Read the model definition and answer for the solid it produces. Units are mm, in the model's axes. Give positions to 0.01 mm unless a question says otherwise; leave off trailing zeros. Write each loop counter-clockwise with the first axis right and the second up, starting at its lowest first coordinate (ties: lowest second). Pieces come first, ordered by that corner, then holes. Notation, with made-up numbers: (71, 32) -> (87, 32) arc R21 cw to (87, 61) -> close; hole circle Ø3 at (46.5, 14.5). An arc over 180 degrees is marked (long way). Use a Markdown table: item, result.
from build123d import *

# Parameters (mm, degrees)
MAIN_PROFILE_SKETCH_W = 70
MAIN_PROFILE_SKETCH_H = 106
MAIN_PROFILE_SKETCH_R = 1.7
MAIN_EXTRUSION_DEPTH  = 3


with BuildPart() as part:
    # Main Profile Sketch → Main Extrusion (new body)
    with BuildSketch(Plane.XY.offset(88)):
        with Locations((-203, 0)):
            Rectangle(MAIN_PROFILE_SKETCH_W, MAIN_PROFILE_SKETCH_H)
        with Locations((-234, -51)):
            Circle(MAIN_PROFILE_SKETCH_R, mode=Mode.SUBTRACT)
        with Locations((-221, -39)):
            Circle(MAIN_PROFILE_SKETCH_R, mode=Mode.SUBTRACT)
        with Locations((-221, -25)):
            Circle(MAIN_PROFILE_SKETCH_R, mode=Mode.SUBTRACT)
        with Locations((-224, -5)):
            Circle(MAIN_PROFILE_SKETCH_R, mode=Mode.SUBTRACT)
        with Locations((-210, -5)):
            Circle(MAIN_PROFILE_SKETCH_R, mode=Mode.SUBTRACT)
        with Locations((-172, -51)):
            Circle(MAIN_PROFILE_SKETCH_R, mode=Mode.SUBTRACT)
        with Locations((-185, -39)):
            Circle(MAIN_PROFILE_SKETCH_R, mode=Mode.SUBTRACT)
        with Locations((-190, -11)):
            Circle(MAIN_PROFILE_SKETCH_R, mode=Mode.SUBTRACT)
        with Locations((-185, -25)):
            Circle(MAIN_PROFILE_SKETCH_R, mode=Mode.SUBTRACT)
        with Locations((-224, 5)):
            Circle(MAIN_PROFILE_SKETCH_R, mode=Mode.SUBTRACT)
        with Locations((-210, 5)):
            Circle(MAIN_PROFILE_SKETCH_R, mode=Mode.SUBTRACT)
        with Locations((-234, 51)):
            Circle(MAIN_PROFILE_SKETCH_R, mode=Mode.SUBTRACT)
        with Locations((-190, 11)):
            Circle(MAIN_PROFILE_SKETCH_R, mode=Mode.SUBTRACT)
        with Locations((-203, 18)):
            Circle(MAIN_PROFILE_SKETCH_R, mode=Mode.SUBTRACT)
        with Locations((-203, 40)):
            Circle(MAIN_PROFILE_SKETCH_R, mode=Mode.SUBTRACT)
        with Locations((-172, 51)):
            Circle(MAIN_PROFILE_SKETCH_R, mode=Mode.SUBTRACT)
    extrude(amount=-MAIN_EXTRUSION_DEPTH)


solid = part.part
Item 1: Straight lines are drawn through the part: line 1 along Y through (x, z) = (-224, 86.7); line 2 along Y through (x, z) = (-172, 86.2); line 3 along X through (y, z) = (-38, 86.9). For each, find the intervals that lie inside material, in ascending order. Write a range as [from, to].
Return value:
| item | result |
|---|---|
| line 1 | [-53, -6.7], [-3.3, 3.3], [6.7, 53] |
| line 2 | [-53, -52.7], [-49.3, 49.3], [52.7, 53] |
| line 3 | [-238, -222.37], [-219.63, -186.37], [-183.63, -168] |
Item 2: A cutting plane is placed at B-B (x = -185). Give the vertices of the cut face in (y, z), then the cut area to 3 significant figures.
Return value:
| item | result |
|---|---|
| outline | (-53, 85) -> (-40.7, 85) -> (-40.7, 88) -> (-53, 88) -> close; (-37.3, 85) -> (-26.7, 85) -> (-26.7, 88) -> (-37.3, 88) -> close; (-23.3, 85) -> (53, 85) -> (53, 88) -> (-23.3, 88) -> close |
| area | 298 mm^2 |
Item 3: A cutting plane is placed at D-D (z = 87.3). Count the separate pieces of the cut face and the enclosed holes in it, then the cut area to 3 significant figures.
Return value:
| item | result |
|---|---|
| separate pieces | 1 |
| enclosed holes | 16 |
| area | 7,270 mm^2 |
Item 4: For a pull along X with two mould halves and no side action, classify faces 1 (the face through (-238, -1, 87)), 2 (the face through (-201.43, 39.35, 86.52)), 3 (the face through (-203, 1, 88)) as +X half, -X half, draft (parallel to the pull), parting line (faces both ways), or undercut.
Return value:
| item | result |
|---|---|
| face 1 | -X half |
| face 2 | undercut |
| face 3 | draft |
Item 5: A cutting plane is placed at A-A (y = 51). Give the vertices of the cut face in (x, z), then the cut area to 3 significant figures.
Return value:
| item | result |
|---|---|
| outline | (-238, 85) -> (-235.7, 85) -> (-235.7, 88) -> (-238, 88) -> close; (-232.3, 85) -> (-173.7, 85) -> (-173.7, 88) -> (-232.3, 88) -> close; (-170.3, 85) -> (-168, 85) -> (-168, 88) -> (-170.3, 88) -> close |
| area | 190 mm^2 |
Item 6: A cutting plane is placed at C-C (y = 40). Give the vertices of the cut face in (x, z).
Return value:
| item | result |
|---|---|
| outline | (-238, 85) -> (-204.7, 85) -> (-204.7, 88) -> (-238, 88) -> close; (-201.3, 85) -> (-168, 85) -> (-168, 88) -> (-201.3, 88) -> close |
Item 7: This flat-tipped pin is pushed along its axis until it touches: P1, Ø5.5, axis at x = -234, y = 51, coming from the -Z side. Where does it stop, or does it pass through?
Return value:
| item | result |
|---|---|
| P1 | z = 85 |
